Part model, mm, in its own coordinate system. Give positions to 0.01 mm unless a question says otherwise; leave off trailing zeros. Order: outer loops, then holes, each group sorted by start corner. A loop starts at its lowest first (then second) coordinate and runs counter-clockwise, first axis right, second up. Notation, with made-up numbers: M -14.5,75 L 17.5,75 A23 cw 17.5,108 Z; hole C 32.25,38.5 d1. An arc over 180 degrees is marked long. Return JSON: item names as keys, results as strings.
from build123d import *

# Parameters (mm, degrees)
SKETCH3_W           = 203.2
SKETCH3_H           = 6.35
BOSS_EXTRUDE1_DEPTH = 152.4
SKETCH5_R           = 1.65
SKETCH5_R_2         = 1.650000002
CUT_EXTRUDE1_DEPTH  = 25400
SKETCH7_R           = 3.52552
CUT_EXTRUDE2_DEPTH  = 2.79908
SKETCH8_R           = 19.05
CUT_EXTRUDE3_DEPTH  = 184.272045059


with BuildPart() as part:
    # Sketch3 → Boss-Extrude1 (new, symmetric)
    with BuildSketch(Plane.XY):
        Rectangle(SKETCH3_W, SKETCH3_H)
    extrude(amount=BOSS_EXTRUDE1_DEPTH, both=True)

    # Sketch5 → Cut-Extrude1 (cut)
    with BuildSketch(Plane(origin=(0, 3.175, 0), x_dir=(1, 0, 0), z_dir=(0, 1, 0))):
        with Locations(Location((7.746566692, 112.45, 0), (0, 0, 270))):
            Circle(SKETCH5_R)
        with Locations(Location((-7.745366692, 112.45, 0), (0, 0, 270))):
            Circle(SKETCH5_R_2)
        with Locations(Location((0.0006, 112.45, 0), (0, 0, 270))):
            Circle(SKETCH5_R)
    extrude(amount=-CUT_EXTRUDE1_DEPTH, mode=Mode.SUBTRACT)

    # Sketch7 → Cut-Extrude2 (cut)
    with BuildSketch(Plane(origin=(0, -3.175, 0), x_dir=(1, 0, 0), z_dir=(0, 1, 0))):
        with Locations(Location((7.746566692, 112.45, 0), (0, 0, 270))):
            Circle(SKETCH7_R)
        with Locations(Location((0.0006, 112.45, 0), (0, 0, 270))):
            Circle(SKETCH7_R)
        with Locations(Location((-7.745366692, 112.45, 0), (0, 0, 270))):
            Circle(SKETCH7_R)
    extrude(amount=CUT_EXTRUDE2_DEPTH, mode=Mode.SUBTRACT)

    # Sketch8 → Cut-Extrude3 (cut, through all)
    with BuildSketch(Plane(origin=(0, 3.175, 0), x_dir=(1, 0, 0), z_dir=(0, 1, 0))):
        with Locations(Location((0, -39.38524, 0), (0, 0, 270))):
            Circle(SKETCH8_R)
    extrude(amount=-CUT_EXTRUDE3_DEPTH, mode=Mode.SUBTRACT)


solid = part.part
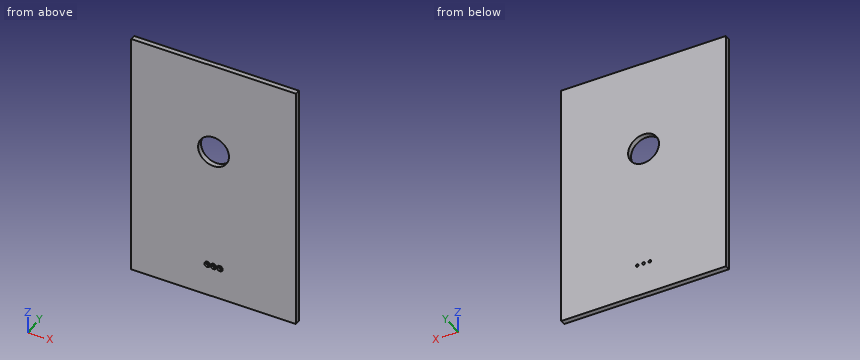
Q1. Probe line 1 along X through (y, z) = (1.55, -112.45); line 2 along X through (y, z) = (-1.8, -112.45); line 3 along X through (y, z) = (2.75, 39). List the from-to ranges inside material, lowest first.
Established:
{"line 1": "x = -101.6 to -9.4, -6.1 to -1.65, 1.65 to 6.1, 9.4 to 101.6", "line 2": "x = -101.6 to -11.27, -4.22 to -3.52, 3.53 to 4.22, 11.27 to 101.6", "line 3": "x = -101.6 to -19.05, 19.05 to 101.6"}
Q2. Pin check, flat tips, straight feed: pin 1 (2 mm diameter, centred on x = 8.5, z = -113.5, fed in from -Y); pin 2 (3 mm diameter, centred on x = 7.75, z = -112.45, fed in from -Y). Stop position of each tip, or through.
Established:
{"pin 1": "stops at y = -0.38", "pin 2": "passes through"}
Q3. Band-saw the part on A-A (y = 1.75). Give the cut face in (x, z), then the cut area to 3 significant figures.
Established:
{"outline": "M -101.6,-152.4 L 101.6,-152.4 L 101.6,152.4 L -101.6,152.4 Z; hole C 0,39.39 d38.1; hole C -7.75,-112.45 d3.3; hole C 0,-112.45 d3.3; hole C 7.75,-112.45 d3.3", "area": "60,800 mm²"}
